from build123d import *

# Parameters (mm, degrees)
SKETCH_R     = 15
SKETCH_R_2   = 12
PAD_DEPTH    = 20
SKETCH001_W  = 20
SKETCH001_H  = 45
PAD001_DEPTH = 3
SKETCH002_R  = 1.5
POCKET_DEPTH = 5
FILLET_R     = 4


with BuildPart() as part:
    # Sketch → Pad (new body)
    with BuildSketch(Plane.YZ):
        Circle(SKETCH_R)
        Circle(SKETCH_R_2, mode=Mode.SUBTRACT)
    extrude(amount=PAD_DEPTH)

    # Sketch001 (on DatumPlane) → Pad001 (join)
    with BuildSketch(Plane.XY.offset(17)):
        with Locations((10.021344, 0)):
            Rectangle(SKETCH001_W, SKETCH001_H)
    extrude(amount=-PAD001_DEPTH)

    # Sketch002 (on Face10 of Pad001) → Pocket (cut)
    with BuildSketch(Plane(origin=(0, 0, 17), x_dir=(0, -1, 0), z_dir=(0, 0, 1))):
        with Locations((-20, 10)):
            Circle(SKETCH002_R)
        with Locations((20, 10)):
            Circle(SKETCH002_R)
    extrude(amount=-POCKET_DEPTH, mode=Mode.SUBTRACT)

    # Fillet
    fillet_edges = [part.edges().sort_by_distance(p)[0] for p in [
        (10.010672, -5.385165, 14),
        (10.010672, 5.385165, 14),
    ]]
    fillet(fillet_edges, radius=FILLET_R)


solid = part.part
Input: part model. Units: mm. Frame: model coordinates. Give positions to 0.01 mm unless a question says otherwise; leave off trailing zeros. Order: outer loops, then holes, each group sorted by start corner. A loop starts at its lowest first (then second) coordinate and runs counter-clockwise, first axis right, second up. Notation, with made-up numbers: (61, 65) -> (71, 65) arc R18 cw to (71, 71) -> close; hole circle Ø11 at (60.5, -27). An arc over 180 degrees is marked (long way). Use one line per item in the form item = value.
1) Section D-D, the plane x = 1.5. Return loops of the section in (y, z), and give its area (3 significant figures).
Response values:
outline = (-22.5, 14) -> (-16.16, 14) arc R4 cw to (-12.75, 7.89) arc R15 ccw (long way) to (12.75, 7.89) arc R4 cw to (16.16, 14) -> (22.5, 14) -> (22.5, 17) -> (-22.5, 17) -> close; hole circle Ø24 at (0, 0)
area = 418 mm^2
2) Line query: probe 1 along X at (y, z) = (20, 14.95); probe 2 along Z at (x, y) = (15, 0.5); probe 3 along X at (y, z) = (12, 1). Output: solid intervals per line, ascending.
Response values:
probe_1 = 0.02 to 8.5, 11.5 to 20.02
probe_2 = -14.99 to -11.99, 11.99 to 17
probe_3 = 0 to 20
3) Section A-A, the plane x = 10. Return loops of the section in (y, z).
Response values:
outline = (-22.5, 14) -> (-21.5, 14) -> (-21.5, 17) -> (-22.5, 17) -> close; (-18.5, 14) -> (-16.16, 14) arc R4 cw to (-12.75, 7.89) arc R15 ccw (long way) to (12.75, 7.89) arc R4 cw to (16.16, 14) -> (18.5, 14) -> (18.5, 17) -> (-18.5, 17) -> close; (21.5, 14) -> (22.5, 14) -> (22.5, 17) -> (21.5, 17) -> close; hole circle Ø24 at (0, 0)
4) Section C-C, the plane z = 0. Return loops of the section in (x, y).
Response values:
outline = (0, -15) -> (20, -15) -> (20, -12) -> (0, -12) -> close; (0, 12) -> (20, 12) -> (20, 15) -> (0, 15) -> close
5) First-contact query: pin 1 Ø8 at (x, z) = (17, 3.5) entering from +Y; pin 2 Ø6 at (x, z) = (13.5, -7.5) entering from +Y; pin 3 Ø4 at (x, z) = (3.5, 0.5) entering from -Y. Flat tips, straight axial feed; report the tip coordinate or a pass-through.
Response values:
pin_1 = 15
pin_2 = 14.31
pin_3 = -15
6) Mould query, pull axis Y, two halves, no side actions, for faces 1 (the flat face through (0, -7, 10)), 2 (the cylindrical face through (10.07, -18.5, 15.52)), 3 (the flat face through (10, -22.5, 16)), 4 (the cylindrical face through (10.07, 21.5, 15.52)). Classes: pulls with the +Y half, pulls with the -Y half, needs draft (parallel to the pull), parting line crosses it, or undercut.
Response values:
face_1 = needs draft
face_2 = undercut
face_3 = pulls with the -Y half
face_4 = undercut
